from build123d import *

# Parameters (mm, degrees)
F0_W     = 5
F0_H     = 30
F1_DEPTH = 20
F3_D     = 5.2
F5_D     = 4.2
F6_SIZE  = 3


with BuildPart() as f1:
    # F0 (on Top) → F1 (new body)
    with BuildSketch(Plane.XY):
        Polygon((6.111111, 39.583333), (6.111111, 32.083333), (66.111111, 32.083333), (66.111111, 39.583333), (47.111111, 39.583333), (42.111111, 39.583333), (30.111111, 39.583333), (25.111111, 39.583333), align=None)
        with Locations((27.611111, 54.583333)):
            Rectangle(F0_W, F0_H)
        with Locations((44.611111, 54.583333)):
            Rectangle(F0_W, F0_H)
    extrude(amount=F1_DEPTH)

    # F3 (through all)
    with Locations(Plane.XZ.offset(-32.083333)):
        with Locations((11.111111, 10), (61.111111, 10)):
            Hole(F3_D / 2)

    # F5 (through all)
    with Locations(Plane(origin=(25.111111, 0, 0), x_dir=(0, -1, 0), z_dir=(-1, 0, 0))):
        with Locations((-60.083333, 10)):
            Hole(F5_D / 2)

    # F6
    f6_edges = [f1.edges().sort_by_distance(p)[0] for p in [
        (27.611111, 69.583333, 20),
        (44.611111, 69.583333, 20),
        (44.611111, 69.583333, 0),
        (27.611111, 69.583333, 0),
        (25.111111, 39.583333, 10),
        (47.111111, 39.583333, 10),
        (42.111111, 39.583333, 10),
        (30.111111, 39.583333, 10),
    ]]
    chamfer(f6_edges, length=F6_SIZE)


solid = f1.part
Could you check a few things on this model? Use its own coordinates, in mm. A direction names the side the tool comes from. Round coordinates to 2 decimals unless told otherwise and drop trailing zeros. Write each loop counter-clockwise with the first axis right and the second up, starting at its lowest first coordinate (ties: lowest second). Pieces come first, ordered by that corner, then holes. Notation, with made-up numbers: (75.5, 67) - (113.5, 67) arc R17 cw to (113.5, 96) - close; hole circle Ø1 at (23, -7). An arc over 180 degrees is marked (long way). Put each result on its own line as item: value. Start each with the question number.
(1) I want a section at A-A, the plane z = 10. Give the number of separate pieces and of enclosed holes in the cut face, plus the area to 3 significant figures.
(2) I want a section at C-C, the plane x = 43. Please give me the cut outline in (y, z), plus the area to 3 significant figures.
(3) I want a section at B-B, the plane y = 49.5. Please give me the cut outline in (x, z), plus the area to 3 significant figures.
(4) Will these pins go through, and if not, where does the flat tip stop? pin 1 (3 mm diameter, centred on x = 11.11, z = 10, fed in from -Y); pin 2 (10 mm diameter, centred on y = 51.5, z = 6.5, fed in from -X); pin 3 (6 mm diameter, centred on y = 52.5, z = 11, fed in from +X); pin 4 (8 mm diameter, centred on x = 16.5, z = 6.5, fed in from +Y).
(5) I need wall thicknesses on probe 1 along X at (y, z) = (51, 1); probe 2 along Y at (x, z) = (39, 11.25); probe 3 along Z at (x, y) = (12, 39). Which ranges of each line are inside material? Lowest first, please.
(6) For faces 1 (the flat face through (31.59, 41.104, 9.86)), 2 (the flat face through (44.576, 68.104, 1.521)), 3 (the flat face through (58, 39.583, 10)), 4 (the flat face through (14, 39.583, 10)), 5 (the flat face through (6.111, 36, 10)), which set-ups out of +Z, -Z, +X, -X, +Y, -Y let a thin tool reach every point of the face, with its end or its side?
(7) I want a section at D-D, the plane x = 12. Please give me the cut outline in (y, z), plus the area to 3 significant figures.
(8) Thinking about a two-plate mould opening in Z: for faces 6 (the flat face through (36, 38, 0)), 7 (the flat face through (66.111, 36, 10)), 8 (the cylindrical face through (58.71, 35.89, 9)), which applies, released by +Z, released by -Z, zero draft, split by the parting line, or undercut?
Here are the results:
1. separate pieces: 5
1. enclosed holes: 0
1. area: 648 mm^2
2. outline: (32.08, 0) - (66.58, 0) - (69.58, 3) - (69.58, 17) - (66.58, 20) - (32.08, 20) - close; hole circle Ø4.2 at (60.08, 10)
2. area: 727 mm^2
3. outline: (25.11, 0) - (30.11, 0) - (30.11, 20) - (25.11, 20) - close; (42.11, 0) - (47.11, 0) - (47.11, 20) - (42.11, 20) - close
3. area: 200 mm^2
4. pin 1: passes through
4. pin 2: stops at x = 25.11
4. pin 3: stops at x = 47.11
4. pin 4: stops at y = 39.58
5. probe 1: x = 25.11 to 30.11, 42.11 to 47.11
5. probe 2: y = 32.08 to 39.58
5. probe 3: z = 0 to 7.56, 12.44 to 20
6. face 1: +Z, -Z, +Y
6. face 2: -Z, +X, -X, +Y
6. face 3: +Z, -Z, +X, +Y
6. face 4: +Z, -Z, -X, +Y
6. face 5: +Z, -Z, -X, +Y, -Y
7. outline: (32.08, 0) - (39.58, 0) - (39.58, 7.56) - (32.08, 7.56) - close; (32.08, 12.44) - (39.58, 12.44) - (39.58, 20) - (32.08, 20) - close
7. area: 113 mm^2
8. face 6: released by -Z
8. face 7: zero draft
8. face 8: undercut
